```python
from build123d import *

# Parameters (mm, degrees)
SKETCH010_R             = 2.75
PAD005_DEPTH            = 35
SKETCH011_W             = 20
SKETCH011_H             = 10
POCKET005_DEPTH         = 167.158509
CHAMFER010_SIZE         = 0.4
SKETCH012_R             = 5.5
POCKET006_DEPTH         = 167.158509
CHAMFER011_SIZE         = 0.4
CHAMFER012_SIZE         = 1
SKETCH013_R             = 2
POCKET007_DEPTH         = 10.001
POCKET007_DEPTH_BACK    = 5.001
CHAMFER013_SIZE         = 1
CHAMFER020_SIZE         = 3
POCKET010_DEPTH         = 15.5
FILLET006_R             = 5
BODY004_PLACEMENT_ANGLE = 90


with BuildPart() as part:
    # Sketch010 → Pad005 (new body, symmetric)
    with BuildSketch(Plane.XY):
        with BuildLine():
            ThreePointArc((5, 0), (3.535534, 3.535534), (0, 5))
            Line((0, 5), (-10, 3))
            Line((-10, 3), (-10, 0))
            Line((-10, 0), (-5, 0))
            Line((-5, 0), (-5, -20))
            Line((-5, -20), (5, -20))
            Line((5, -20), (5, 0))
        make_face()
        Circle(SKETCH010_R, mode=Mode.SUBTRACT)
    extrude(amount=PAD005_DEPTH, both=True)

    # Sketch011 → Pocket005 (cut, through all)
    with BuildSketch(Plane.XY.offset(19.5)):
        with Locations((-5, 0)):
            Rectangle(SKETCH011_W, SKETCH011_H)
    pocket005 = extrude(amount=POCKET005_DEPTH, mode=Mode.SUBTRACT)

    # Mirrored: Pocket005 across XY
    add(pocket005.mirror(Plane.XY), mode=Mode.SUBTRACT)

    # Chamfer010
    chamfer010_edges = [part.edges().sort_by_distance(p)[0] for p in [
        (-10, 3, 0),
        (-10, 0, 0),
    ]]
    chamfer(chamfer010_edges, length=CHAMFER010_SIZE)

    # Sketch012 (on Face12 of Chamfer010) → Pocket006 (cut, through all)
    with BuildSketch(Plane.XY.offset(19.5)):
        Circle(SKETCH012_R)
    pocket006 = extrude(amount=POCKET006_DEPTH, mode=Mode.SUBTRACT)

    # Mirrored001: Pocket006 across XY
    add(pocket006.mirror(Plane.XY), mode=Mode.SUBTRACT)

    # Chamfer011
    chamfer011_edges = [part.edges().sort_by_distance(p)[0] for p in [
        (-2.291288, -5, -27.25),
        (2.291288, -5, -27.25),
        (2.291288, -5, 27.25),
        (-2.291288, -5, 27.25),
    ]]
    chamfer(chamfer011_edges, length=CHAMFER011_SIZE)

    # Chamfer012
    chamfer012_edges = [part.edges().sort_by_distance(p)[0] for p in [
        (-5, -5, 27.25),
        (5, -5, 27.25),
        (5, -5, -27.25),
        (-5, -5, -27.25),
        (-5, -20, 0),
        (5, -20, 0),
    ]]
    chamfer(chamfer012_edges, length=CHAMFER012_SIZE)

    # Sketch013 → Pocket007 (cut, two sides)
    with BuildSketch(Plane.YZ) as pocket007_sk:
        with Locations((-13, 28)):
            Circle(SKETCH013_R)
        with Locations((-13, -28)):
            Circle(SKETCH013_R)
    extrude(amount=-POCKET007_DEPTH, mode=Mode.SUBTRACT)
    extrude(pocket007_sk.sketch, amount=POCKET007_DEPTH_BACK, mode=Mode.SUBTRACT)

    # Chamfer013
    chamfer013_edges = [part.edges().sort_by_distance(p)[0] for p in [
        (-5, -15, -28),
        (-5, -15, 28),
    ]]
    chamfer(chamfer013_edges, length=CHAMFER013_SIZE)

    # Chamfer020
    chamfer020_edges = [part.edges().sort_by_distance(p)[0] for p in [
        (5, -15, -28),
        (5, -15, 28),
    ]]
    chamfer(chamfer020_edges, length=CHAMFER020_SIZE)

    # Sketch017 (on Face9 of Chamfer020) → Pocket010 (cut)
    with BuildSketch(Plane.XY.offset(35)):
        Polygon((5, -5), (1, -5), (5, -9), align=None)
    pocket010 = extrude(amount=-POCKET010_DEPTH, mode=Mode.SUBTRACT)

    # Mirrored002: Pocket010 across XY
    add(pocket010.mirror(Plane.XY), mode=Mode.SUBTRACT)

    # Fillet006
    fillet006_edges = [part.edges().sort_by_distance(p)[0] for p in [
        (1.335416, -5.335416, 27.25),
        (1.335416, -5.335416, -27.25),
    ]]
    fillet(fillet006_edges, radius=FILLET006_R)


with BuildPart() as part_1:
    # Body004 placement: moved
    add(part.part.rotate(Axis((0, 0, 0), (0, 0, 1)), BODY004_PLACEMENT_ANGLE))


solid = part_1.part
```
Input: part model. Units: mm. Frame: model coordinates. A direction names the side the tool comes from. Give positions to 0.01 mm unless a question says otherwise; leave off trailing zeros. Write each loop counter-clockwise with the first axis right and the second up, starting at its lowest first coordinate (ties: lowest second). Pieces come first, ordered by that corner, then holes. Notation, with made-up numbers: (80.5, -7) - (90.5, -7) arc R6 cw to (90.5, -3) - close; hole circle Ø11 at (81.25, 61). An arc over 180 degrees is marked (long way). Write item = value, one per line. Start each with the question number.
1. Section query C-C, the plane z = 0. Output: boundary loops of the cut face in (x, y), then the cut area to 3 significant figures.
2. Section query B-B, the plane x = 13. Output: boundary loops of the cut face in (y, z), then the cut area to 3 significant figures.
3. Access query for faces 4 (the flat face through (0, -7, 0)), 5 (the flat face through (8, 4, -27)), 6 (the flat face through (5, -3, 27)), 7 (the flat face through (8, 4, 27)), 8 (the flat face through (-2, -10, 0)). Directions: +Z, -Z, +X, -X, +Y, -Y. A direction counts if a zero-diameter tool reaches every point of the face in a straight line with its end or side. Return the directions, or none.
4. Ray query, L1, parallel to Z at x = 13, y = -1.5; L2, parallel to Z at x = 12, y = -1; L3, parallel to Z at x = -0.5, y = -5. Return the intervals inside material, ascending.
5. Mould query, pull axis X, two halves, no side actions, for faces 1 (the flat face through (12, 0, 35)), 2 (the flat face through (5, -3, -27)), 3 (the conical face through (15.2, 2.2, 27.9)). Classes: released by +X, released by -X, zero draft, split by the parting line, or undercut.
6. First-contact query: pin 1 Ø0.7 at (y, z) = (-3.5, -29.5) entering from -X; pin 2 Ø10 at (x, z) = (2.5, 6) entering from -Y; pin 3 Ø15 at (x, z) = (9, -8.5) entering from -Y; pin 4 Ø3.5 at (x, z) = (13, 28) entering from -Y. Flat tips, straight axial feed; report the tip coordinate or a pass-through.
7. Section query A-A, the plane z = -28. Output: boundary loops of the cut face in (x, y).
Check sheet entries:
q1.outline = (-5, 0) - (-3.08, -9.61) - (-2.6, -10) - (-0.4, -10) - (0, -9.6) - (0, -5) - (19, -5) - (20, -4) - (20, 4) - (19, 5) - (0, 5) arc R5 ccw to start; hole circle Ø5.5 at (0, 0)
q1.area = 235 mm2
q2.outline = (-5, -35) - (5, -35) - (5, -33) - (2, -30) - (-4, -30) - (-5, -31) - close; (-5, -25) - (-4, -26) - (2, -26) - (5, -23) - (5, 23) - (2, 26) - (-4, 26) - (-5, 25) - close; (-5, 31) - (-4, 30) - (2, 30) - (5, 33) - (5, 35) - (-5, 35) - close
q2.area = 600 mm2
q3.face_4 = +Z, -Z, +X, -Y
q3.face_5 = -Z, -X, +Y
q3.face_6 = +Z, -X, +Y, -Y
q3.face_7 = +Z, -X, +Y
q3.face_8 = +Z, -Z, +X, -X, -Y
q4.L1 = -35 to -30, -26 to 26, 30 to 35
q4.L2 = -35 to -29.73, -26.27 to 26.27, 29.73 to 35
q4.L3 = -19.5 to 19.5
q5.face_1 = zero draft
q5.face_2 = released by -X
q5.face_3 = undercut
q6.pin_1 = 5
q6.pin_2 = -10
q6.pin_3 = -5
q6.pin_4 = through
q7.outline = (5, -4) - (6, -5) - (10, -5) - (11, -4) - (11, 2) - (8.5, 4.5) - (6.95, 2.95) arc R5 ccw to (5.49, -0.31) arc R5.5 cw to (5.15, -1.92) - (5, -2.69) - close; (15, -4) - (16, -5) - (19, -5) - (20, -4) - (20, 4) - (19, 5) - (18, 5) - (15, 2) - close
